```python
from build123d import *

# Parameters (mm, degrees)
SALIENTE_EXTRUIR1_DEPTH = 13
CROQUIS2_W              = 7
CROQUIS2_H              = 20
CORTAR_EXTRUIR1_DEPTH   = 7.6
CROQUIS3_W              = 3
CROQUIS3_H              = 5.399999618
CROQUIS3_H_2            = 5.399999619
CORTAR_EXTRUIR2_DEPTH   = 5.4
CROQUIS4_R              = 1
CORTAR_EXTRUIR3_DEPTH   = 10.4
CORTAR_EXTRUIR4_DEPTH   = 32.4
CROQUIS6_W              = 66.642206308
CROQUIS6_H              = 2.2
CORTAR_EXTRUIR5_DEPTH   = 35


with BuildPart() as part:
    # Croquis1 → Saliente-Extruir1 (new body)
    with BuildSketch(Plane(origin=(0, 0, 0), x_dir=(1, 0, 0), z_dir=(0, 1, 0))):
        Polygon((-29.00453802, -14.532941153), (-29.00453802, -9.132941534), (22.99546198, -9.132941534), (22.99546198, 10.867058466), (-29.00453802, 10.867058466), (-29.00453802, 16.267058084), (23.998794118, 16.267058084), (29.99546198, 12.804880808), (29.99546198, -11.070763876), (23.998794118, -14.532941153), align=None)
    extrude(amount=SALIENTE_EXTRUIR1_DEPTH)

    # Croquis2 → Cortar-Extruir1 (cut)
    with BuildSketch(Plane(origin=(0, 13, 0), x_dir=(1, 0, 0), z_dir=(0, 1, 0))):
        with Locations((26.49546198, 0.867058466)):
            Rectangle(CROQUIS2_W, CROQUIS2_H)
    extrude(amount=-CORTAR_EXTRUIR1_DEPTH, mode=Mode.SUBTRACT)

    # Croquis3 → Cortar-Extruir2 (cut)
    with BuildSketch(Plane(origin=(0, 13, 0), x_dir=(1, 0, 0), z_dir=(0, 1, 0))):
        with Locations((-27.50453802, 13.567058275)):
            Rectangle(CROQUIS3_W, CROQUIS3_H)
        with Locations((-27.50453802, -11.832941343)):
            Rectangle(CROQUIS3_W, CROQUIS3_H_2)
    extrude(amount=-CORTAR_EXTRUIR2_DEPTH, mode=Mode.SUBTRACT)

    # Croquis4 → Cortar-Extruir3 (cut)
    with BuildSketch(Plane(origin=(0, 5.4, 0), x_dir=(1, 0, 0), z_dir=(0, 1, 0))):
        with Locations((26.49546198, 5.867058466)):
            Circle(CROQUIS4_R)
        with Locations((26.49546198, -4.132941534)):
            Circle(CROQUIS4_R)
    extrude(amount=-CORTAR_EXTRUIR3_DEPTH, mode=Mode.SUBTRACT)

    # Croquis5 → Cortar-Extruir4 (cut)
    with BuildSketch(Plane.XY.offset(14.532941153)):
        Polygon((28.23546198, 0), (29.99546198, 3.04), (29.99546198, 0), align=None)
    extrude(amount=-CORTAR_EXTRUIR4_DEPTH, mode=Mode.SUBTRACT)

    # Croquis6 → Cortar-Extruir5 (cut)
    with BuildSketch(Plane(origin=(0, 0, -16.267058084), x_dir=(-1, 0, 0), z_dir=(0, 0, -1))):
        with Locations((-4.316565134, 1.1)):
            Rectangle(CROQUIS6_W, CROQUIS6_H)
    extrude(amount=-CORTAR_EXTRUIR5_DEPTH, mode=Mode.SUBTRACT)


solid = part.part
```
Geometry check sheet. Reference: the model listing, model coordinates, mm. A direction names the side the tool comes from. Round coordinates to 2 decimals unless told otherwise and drop trailing zeros. Order: outer loops, then holes, each group sorted by start corner. A loop starts at its lowest first (then second) coordinate and runs counter-clockwise, first axis right, second up. Notation, with made-up numbers: (12.25, -7) - (30.25, -7) arc R19 ccw to (30.25, -1) - close; hole circle Ø8 at (52.5, 67.5). An arc over 180 degrees is marked (long way). Use a Markdown table: item, result. Add a question column.
1) Section check B-B (x = 20). Record the cut outline in (y, z), then the cut area to 3 significant figures.
2) Mould release check, pull along Z, two halves, no side actions. Record for faces 1 (the cylindrical face through (27.45, 3.82, 3.83)), 2 (the flat face through (-28, 7.6, -14)), 3 (the flat face through (-3, 8, -16.267)): released by +Z, released by -Z, zero draft, split by the parting line, or undercut.
3) Section check D-D (y = 6.25). Record the cut outline in (x, z), then the cut area to 3 significant figures.
4) Section check A-A (y = 11). Record the cut outline in (x, z).
5) Thickness scan on line 1 along Z through (x, y) = (-24, 12.5); line 2 along X through (y, z) = (8.25, 10); line 3 along Y through (x, z) = (24, 7). Record the ranges inside material, lowest first.
6) Gauge pin test, flat ends, axial feed: P1, Ø2.5, axis at y = 10.5, z = -14.5, coming from the -X side; P2, Ø3.5, axis at x = 28, z = 3.5, coming from the +Y side; P3, Ø2.5, axis at x = -28, z = 12.5, coming from the +Y side; P4, Ø1, axis at y = 6.5, z = -2, coming from the +X side. Record the tip position at first contact, or that the pin passes through.
7) Section check C-C (z = -12). Record the cut outline in (x, y), then the cut area to 3 significant figures.
8) Set-up check for faces 4 (the flat face through (-26.005, 10, -14)), 5 (the flat face through (26, 5.4, -1)), 6 (the flat face through (26.955, 7.524, -14.56)): record each of +Z, -Z, +X, -X, +Y, -Y from which the full face is reachable in a straight line by a thin tool's end or side.
Established:
| question | item | result |
|---|---|---|
| 1 | outline | (2.2, -16.27) - (13, -16.27) - (13, -10.87) - (2.2, -10.87) - close; (2.2, 9.13) - (13, 9.13) - (13, 14.53) - (2.2, 14.53) - close |
| 1 | area | 117 mm2 |
| 2 | face 1 | undercut |
| 2 | face 2 | zero draft |
| 2 | face 3 | released by -Z |
| 3 | outline | (-29, -16.27) - (24, -16.27) - (30, -12.8) - (30, -10.87) - (-29, -10.87) - close; (-29, 9.13) - (30, 9.13) - (30, 11.07) - (24, 14.53) - (-29, 14.53) - close |
| 3 | area | 616 mm2 |
| 4 | outline | (-26, -16.27) - (24, -16.27) - (30, -12.8) - (30, -10.87) - (-26, -10.87) - close; (-26, 9.13) - (30, 9.13) - (30, 11.07) - (24, 14.53) - (-26, 14.53) - close |
| 5 | line 1 | -16.27 to -10.87, 9.13 to 14.53 |
| 5 | line 2 | -26 to 30 |
| 5 | line 3 | 2.2 to 5.4 |
| 6 | P1 | x = -26 |
| 6 | P2 | y = 5.4 |
| 6 | P3 | y = 7.6 |
| 6 | P4 | through |
| 7 | outline | (-29, 2.2) - (29.51, 2.2) - (30, 3.04) - (30, 13) - (-26, 13) - (-26, 7.6) - (-29, 7.6) - close |
| 7 | area | 621 mm2 |
| 8 | face 4 | +Z, -Z, -X, +Y |
| 8 | face 5 | +X, -X, +Y |
| 8 | face 6 | -Z, +X, +Y, -Y |
